Input: part model. Units: mm. Frame: model coordinates. A direction names the side the tool comes from. Round coordinates to 2 decimals unless told otherwise and drop trailing zeros. Write each loop counter-clockwise with the first axis right and the second up, starting at its lowest first coordinate (ties: lowest second). Pieces come first, ordered by that corner, then holes. Notation, with made-up numbers: (40.25, 10) - (94.25, 10) arc R23 ccw to (94.25, 45) - close; hole circle Ø6 at (33, -24). An arc over 180 degrees is marked (long way). One line per item, written item: value. Start each with the question number.
```python
from build123d import *

# Parameters (mm, degrees)
SKETCH1_R           = 6.5
BOSS_EXTRUDE1_DEPTH = 42.5
SKETCH2_R           = 8
BOSS_EXTRUDE2_DEPTH = 2
SKETCH3_R           = 6.5
SKETCH3_R_2         = 4.5
CUT_EXTRUDE1_DEPTH  = 1


with BuildPart() as part:
    # Sketch1 → Boss-Extrude1 (new body, symmetric)
    with BuildSketch(Plane.XY):
        Circle(SKETCH1_R)
    extrude(amount=BOSS_EXTRUDE1_DEPTH, both=True)

    # Sketch2 → Boss-Extrude2 (add)
    with BuildSketch(Plane.XY.offset(-12.5)):
        Circle(SKETCH2_R)
    extrude(amount=BOSS_EXTRUDE2_DEPTH)

    # Sketch3 → Cut-Extrude1 (cut)
    with BuildSketch(Plane(origin=(0, 0, -40.5), x_dir=(-1, 0, 0), z_dir=(0, 0, -1))):
        Circle(SKETCH3_R)
        Circle(SKETCH3_R_2, mode=Mode.SUBTRACT)
    cut_extrude1 = extrude(amount=-CUT_EXTRUDE1_DEPTH, mode=Mode.SUBTRACT)

    # Mirror1: Cut-Extrude1 across plane
    add(cut_extrude1.mirror(Plane.XY), mode=Mode.SUBTRACT)


solid = part.part
```
Q1. Cut plane A-A, the plane x = 0. Output: boundary loops of the cut face in (y, z), and give its area (3 significant figures).
Q2. Access query for faces 4 (the flat face through (0, 7, -10.5)), 5 (the cylindrical face through (-5.158, -3.955, -41.486)), 6 (the flat face through (4.42, 1.54, -39.5)), 7 (the flat face through (0, 0, -42.5)). Directions: +Z, -Z, +X, -X, +Y, -Y. A direction counts if a zero-diameter tool reaches every point of the face in a straight line with its end or side. Return the directions, or none.
Q3. Material intervals for probe 1 along Z at (x, y) = (-3.5, -4); probe 2 along X at (y, z) = (0, 0.5); probe 3 along Z at (x, y) = (-2.5, -7.5), sorted ascending. Write a range as from..to.
Q4. Cut plane C-C, the plane z = 20. Output: boundary loops of the cut face in (x, y).
Q5. Contact query for flat-ended pins moving along their axis: pin 1 Ø3 at (y, z) = (4, 30) entering from +X; pin 2 Ø4 at (y, z) = (-5.5, 27) entering from +X; pin 3 Ø2 at (x, z) = (6, 1) entering from +Y. Output: stop coordinate, or through.
Q6. Pull-direction query (Z, two-part tool) for faces 1 (the flat face through (0, 0, 42.5)), 2 (the cylindrical face through (-1.73, -7.81, -11.51)), 3 (the flat face through (4.42, 1.54, -40.5)); classes: pulls with the +Z half, pulls with the -Z half, needs draft (parallel to the pull), parting line crosses it, or undercut.
A:
1. outline: (-8, -12.5) - (-6.5, -12.5) - (-6.5, -39.5) - (-4.5, -39.5) - (-4.5, -40.5) - (-6.5, -40.5) - (-6.5, -42.5) - (6.5, -42.5) - (6.5, -40.5) - (4.5, -40.5) - (4.5, -39.5) - (6.5, -39.5) - (6.5, -12.5) - (8, -12.5) - (8, -10.5) - (6.5, -10.5) - (6.5, 39.5) - (4.5, 39.5) - (4.5, 40.5) - (6.5, 40.5) - (6.5, 42.5) - (-6.5, 42.5) - (-6.5, 40.5) - (-4.5, 40.5) - (-4.5, 39.5) - (-6.5, 39.5) - (-6.5, -10.5) - (-8, -10.5) - close
1. area: 1,100 mm²
2. face 4: +Z
2. face 5: -Z
2. face 6: none
2. face 7: -Z, +X, -X, +Y, -Y
3. probe 1: z = -42.5..-40.5, -39.5..39.5, 40.5..42.5
3. probe 2: x = -6.5..6.5
3. probe 3: z = -12.5..-10.5
4. outline: circle Ø13 at (0, 0)
5. pin 1: stops at x = 6
5. pin 2: stops at x = 5.48
5. pin 3: stops at y = 4.15
6. face 1: pulls with the +Z half
6. face 2: needs draft
6. face 3: undercut
